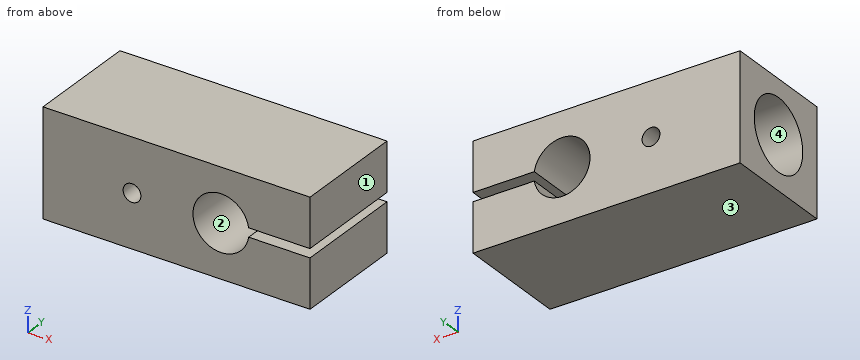
from build123d import *

# Parameters (mm, degrees)
SKETCH1_W           = 30
SKETCH1_H           = 12
SKETCH1_R           = 3.15
SKETCH1_R_2         = 1
BOSS_EXTRUDE1_DEPTH = 12.7
SKETCH2_R           = 4
CUT_EXTRUDE1_DEPTH  = 10
SKETCH3_W           = 6.889935692
SKETCH3_H           = 1
CUT_EXTRUDE2_DEPTH  = 25.439517314


with BuildPart() as part:
    # Sketch1 → Boss-Extrude1 (new body)
    with BuildSketch(Plane(origin=(0, 0, 0), x_dir=(1, 0, 0), z_dir=(0, 1, 0))):
        with Locations((-5, 0)):
            Rectangle(SKETCH1_W, SKETCH1_H)
        with Locations(Location((0, 0, 0), (0, 0, 270))):
            Circle(SKETCH1_R, mode=Mode.SUBTRACT)
        with Locations(Location((-10, 0, 0), (0, 0, 270))):
            Circle(SKETCH1_R_2, mode=Mode.SUBTRACT)
    extrude(amount=BOSS_EXTRUDE1_DEPTH)

    # Sketch2 → Cut-Extrude1 (cut)
    with BuildSketch(Plane.ZY.offset(20)):
        with Locations((0, 6.35)):
            Circle(SKETCH2_R)
    extrude(amount=-CUT_EXTRUDE1_DEPTH, mode=Mode.SUBTRACT)

    # Sketch3 → Cut-Extrude2 (cut, through all)
    with BuildSketch(Plane(origin=(0, 12.7, 0), x_dir=(1, 0, 0), z_dir=(0, 1, 0))):
        with Locations((6.555032154, 0)):
            Rectangle(SKETCH3_W, SKETCH3_H)
    extrude(amount=-CUT_EXTRUDE2_DEPTH, mode=Mode.SUBTRACT)


solid = part.part
Verification items for the finished model (mm, model axes). Face numbers are marked on the shaded views. Coordinates: 2 decimals unless noted, no trailing zeros. Order: outer loops, then holes, each group sorted by start corner. A loop starts at its lowest first (then second) coordinate and runs counter-clockwise, first axis right, second up. Notation, with made-up numbers: (69.5, 68.25) -> (94.5, 68.25) arc R32 ccw to (94.5, 97.25) -> close; hole circle Ø8 at (84, 54.25). An arc over 180 degrees is marked (long way). Put each result on its own line as item: value. Start each with the question number.
1. Material ranges on L1, parallel to Y at x = -12, z = 0; L2, parallel to Z at x = -17.5, y = 6.5; L3, parallel to Z at x = 6, y = 4, recorded low to high. Write a range as [from, to].
2. Cross-section at A-A, the plane x = 4.5. Record the boundary of the cut face in (y, z).
3. Cross-section at C-C, the plane x = -16. Record the boundary of the cut face in (y, z), then the cut area to 3 significant figures.
4. Cross-section at D-D, the plane y = 6.35. Record the boundary of the cut face in (x, z).
5. Mould release check, pull along Z, two halves, no side actions. Record for the marked faces 1, 2, 3 and 4: released by +Z, released by -Z, zero draft, split by the parting line, or undercut.
6. Cross-section at B-B, the plane z = 0. Record the boundary of the cut face in (x, y), then the cut area to 3 significant figures.
7. Go/stop test with a flat-tipped pin: pin 1 Ø0.9 at (y, z) = (4.5, -2) entering from -X. Record where the tip stops, or that it passes through.
Computed:
1. L1: [0, 2.35], [10.35, 12.7]
1. L2: [-6, -4], [4, 6]
1. L3: [-6, -0.5], [0.5, 6]
2. outline: (0, -6) -> (12.7, -6) -> (12.7, -0.5) -> (0, -0.5) -> close; (0, 0.5) -> (12.7, 0.5) -> (12.7, 6) -> (0, 6) -> close
3. outline: (0, -6) -> (12.7, -6) -> (12.7, 6) -> (0, 6) -> close; hole circle Ø8 at (6.35, 0)
3. area: 102 mm2
4. outline: (-20, -6) -> (10, -6) -> (10, -0.5) -> (3.11, -0.5) arc R3.15 cw (long way) to (3.11, 0.5) -> (10, 0.5) -> (10, 6) -> (-20, 6) -> (-20, 4) -> (-10, 4) -> (-10, 1) arc R1 cw to (-10, -1) -> (-10, -4) -> (-20, -4) -> close
5. face 1: zero draft
5. face 2: undercut
5. face 3: released by -Z
5. face 4: undercut
6. outline: (-20, 0) -> (-11, 0) -> (-11, 2.35) -> (-20, 2.35) -> close; (-20, 10.35) -> (-11, 10.35) -> (-11, 12.7) -> (-20, 12.7) -> close; (-9, 0) -> (-3.15, 0) -> (-3.15, 12.7) -> (-9, 12.7) -> close
6. area: 117 mm2
7. pin 1: x = -10
